```python
from build123d import *

# Parameters (mm, degrees)
SKETCH1_R           = 10
BOSS_EXTRUDE1_DEPTH = 10
SKETCH2_R           = 1.5
BOSS_EXTRUDE2_DEPTH = 15
CUT_EXTRUDE1_DEPTH  = 8
SKETCH4_R           = 10
BOSS_EXTRUDE3_DEPTH = 10


with BuildPart() as part:
    # Sketch1 → Boss-Extrude1 (new body)
    with BuildSketch(Plane(origin=(0, 0, 0), x_dir=(1, 0, 0), z_dir=(0, 1, 0))):
        Circle(SKETCH1_R)
    extrude(amount=BOSS_EXTRUDE1_DEPTH)

    # Sketch2 → Boss-Extrude2 (add)
    with BuildSketch(Plane(origin=(0, 10, 0), x_dir=(1, 0, 0), z_dir=(0, 1, 0))):
        Circle(SKETCH2_R)
    extrude(amount=BOSS_EXTRUDE2_DEPTH)

    # Sketch3 → Cut-Extrude1 (cut)
    with BuildSketch(Plane.XZ):
        Polygon((7, 0), (3.5, 6.062177826), (-3.5, 6.062177826), (-7, 0), (-3.5, -6.062177826), (3.5, -6.062177826), align=None)
    extrude(amount=-CUT_EXTRUDE1_DEPTH, mode=Mode.SUBTRACT)

    # Sketch4 → Boss-Extrude3 (add)
    with BuildSketch(Plane(origin=(0, 25, 0), x_dir=(1, 0, 0), z_dir=(0, 1, 0))):
        Circle(SKETCH4_R)
    extrude(amount=BOSS_EXTRUDE3_DEPTH)


solid = part.part
```
For this review, take the finished solid that the model builds, in its own axes (mm). A direction names the side the tool comes from. Coordinates: 2 decimals unless noted, no trailing zeros. Order: outer loops, then holes, each group sorted by start corner. A loop starts at its lowest first (then second) coordinate and runs counter-clockwise, first axis right, second up. Notation, with made-up numbers: (38, 35.25) - (61, 35.25) arc R11 cw to (61, 56.25) - close; hole circle Ø9 at (89.5, -1.5). An arc over 180 degrees is marked (long way). Answer as a JSON object with one key per item and string values. Group by question number.
1. We need section D-D on x = 0. State the section outline as (y, z) points, then the cut area to 3 significant figures.
2. We need section A-A on z = -8. State the section outline as (x, y) points.
3. We need section B-B on x = 4.5. State the section outline as (y, z) points.
4. For faces 4 (the flat face through (-5.274, 3.944, -2.989)), 5 (the cylindrical face through (-1.5, 17.4, -0.07)), 6 (the flat face through (0, 35, 0)), list the 3-axis set-ups (+Z, -Z, +X, -X, +Y, -Y) from which the entire face can be reached by the end or side of a thin tool; tool diameter is ignored.
5. For probe 1 along Y at (x, z) = (-1.25, -2.5); probe 2 along Y at (x, z) = (-6.75, 3.75); probe 3 along X at (y, z) = (6, 0), list the stretches that pass through material, from the lowest coordinate up.
6. Clearance check with flat-ended pins moving along their axes: P1, Ø8, axis at x = 7.5, y = 19, coming from the -Z side; P2, Ø2, axis at x = 1.5, y = 5, coming from the +Z side; P3, Ø1.5, axis at x = -1.5, z = 2, coming from the -Y side; P4, Ø8, axis at y = 24, z = -4, coming from the -X side. State where each tip first meets the part, or that it passes through.
7. The part is to be moulded in two halves that separate along Z. For faces 1 (the flat face through (0, 8, 0)), 2 (the flat face through (2, 10, 0)), 3 (the cylindrical face through (-2.17, 4.93, 9.76)), say which applies: pulls with the +Z half, pulls with the -Z half, needs draft (parallel to the pull), parting line crosses it, or undercut.
8. We need section C-C on y = 6. State the section outline as (x, z) points.
Final values:
{
 "1": {"outline": "(0, -10) - (10, -10) - (10, -1.5) - (25, -1.5) - (25, -10) - (35, -10) - (35, 10) - (25, 10) - (25, 1.5) - (10, 1.5) - (10, 10) - (0, 10) - (0, 6.06) - (8, 6.06) - (8, -6.06) - (0, -6.06) - close", "area": "348 mm²"},
 "2": {"outline": "(-6, 0) - (6, 0) - (6, 10) - (-6, 10) - close; (-6, 25) - (6, 25) - (6, 35) - (-6, 35) - close"},
 "3": {"outline": "(0, -8.93) - (10, -8.93) - (10, 8.93) - (0, 8.93) - (0, 4.33) - (8, 4.33) - (8, -4.33) - (0, -4.33) - close; (25, -8.93) - (35, -8.93) - (35, 8.93) - (25, 8.93) - close"},
 "4": {"face 4": "-Y", "face 5": "none", "face 6": "+Z, -Z, +X, -X, +Y"},
 "5": {"probe 1": "8 to 10, 25 to 35", "probe 2": "0 to 10, 25 to 35", "probe 3": "-10 to -7, 7 to 10"},
 "6": {"P1": "through", "P2": "z = 9.99", "P3": "y = 8", "P4": "x = -10"},
 "7": {"face 1": "undercut", "face 2": "needs draft", "face 3": "parting line crosses it"},
 "8": {"outline": "circle Ø20 at (0, 0); hole (-7, 0) - (-3.5, -6.06) - (3.5, -6.06) - (7, 0) - (3.5, 6.06) - (-3.5, 6.06) - close"}
}
